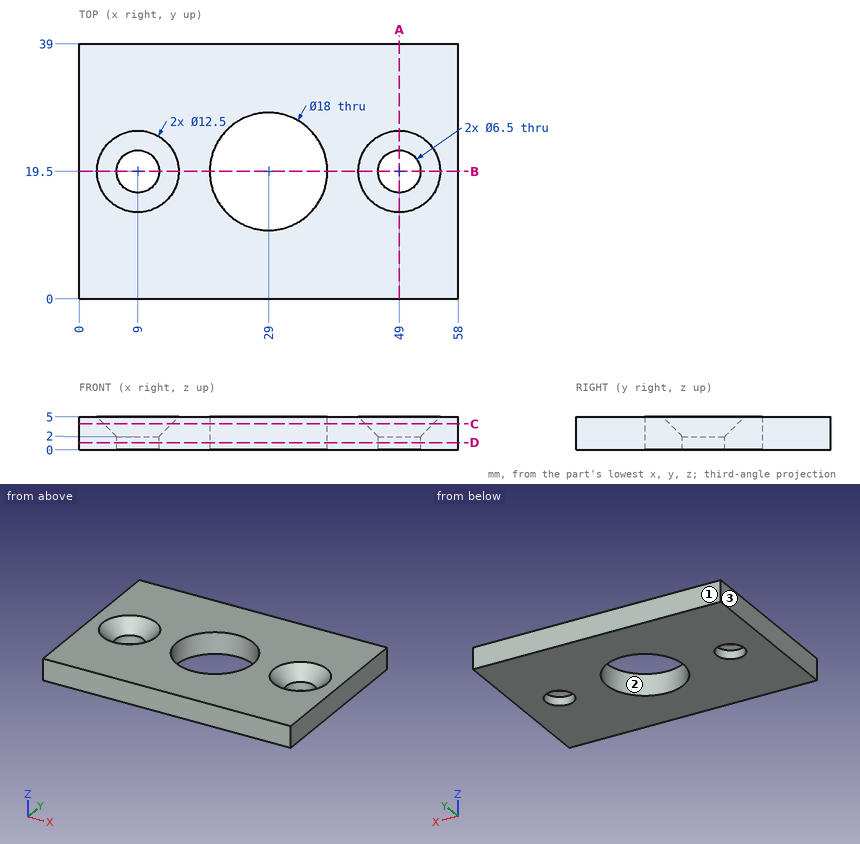
Geometry: see drawing. Coordinates: mm, zero at the bounding-box minimum. Round coordinates to 2 decimals unless told otherwise and drop trailing zeros. Loops run counter-clockwise (first coordinate to the right, second up) from the corner with the lowest first, then second, coordinate; pieces in that order, holes last. Notation, with made-up numbers: (67, 78.25) - (83, 78.25) arc R3 cw to (83, 82.25) - close; hole circle Ø6 at (5, -30). An arc over 180 degrees is marked (long way). Write item = value, one per line. Start each with the question number.
(1) Section query D-D, the plane z = 1.05. Output: boundary loops of the cut face in (x, y), plus the area to 3 significant figures.
(2) Section query A-A, the plane x = 49. Output: boundary loops of the cut face in (y, z), plus the area to 4 significant figures.
(3) Section query C-C, the plane z = 3.95. Output: boundary loops of the cut face in (x, y).
(4) Pull-direction query (Y, two-part tool) for the marked faces 1, 2 and 3; classes: +Y half, -Y half, draft (parallel to the pull), parting line (faces both ways), or undercut.
(5) Pin query (flat end, axial travel): pin 1 (8.5 mm diameter, centred on x = 9, y = 19.5, fed in from +Z). Return the tip coordinate at first contact, or that it passes through.
(6) Ray query, line 1 along Y through (x, z) = (49, 0.85); line 2 along Y through (x, z) = (29, 3.9); line 3 along X through (y, z) = (23, 2). Return the intervals inside material, ascending. Write a range as from..to.
(7) Section query B-B, the plane y = 19.5. Output: boundary loops of the cut face in (x, z).
Conclusion:
q1.outline = (0, 0) - (58, 0) - (58, 39) - (0, 39) - close; hole circle Ø6.5 at (9, 19.5); hole circle Ø18 at (29, 19.5); hole circle Ø6.5 at (49, 19.5)
q1.area = 1,940 mm2
q2.outline = (0, 0) - (16.25, 0) - (16.25, 2) - (13.25, 5) - (0, 5) - close; (22.75, 0) - (39, 0) - (39, 5) - (25.75, 5) - (22.75, 2) - close
q2.area = 153.5 mm2
q3.outline = (0, 0) - (58, 0) - (58, 39) - (0, 39) - close; hole circle Ø10.4 at (9, 19.5); hole circle Ø18 at (29, 19.5); hole circle Ø10.4 at (49, 19.5)
q4.face_1 = +Y half
q4.face_2 = undercut
q4.face_3 = draft
q5.pin_1 = 3
q6.line_1 = 0..16.25, 22.75..39
q6.line_2 = 0..10.5, 28.5..39
q6.line_3 = 0..20.71, 37.29..58
q7.outline = (0, 0) - (5.75, 0) - (5.75, 2) - (2.75, 5) - (0, 5) - close; (12.25, 0) - (20, 0) - (20, 5) - (15.25, 5) - (12.25, 2) - close; (38, 0) - (45.75, 0) - (45.75, 2) - (42.75, 5) - (38, 5) - close; (52.25, 0) - (58, 0) - (58, 5) - (55.25, 5) - (52.25, 2) - close
